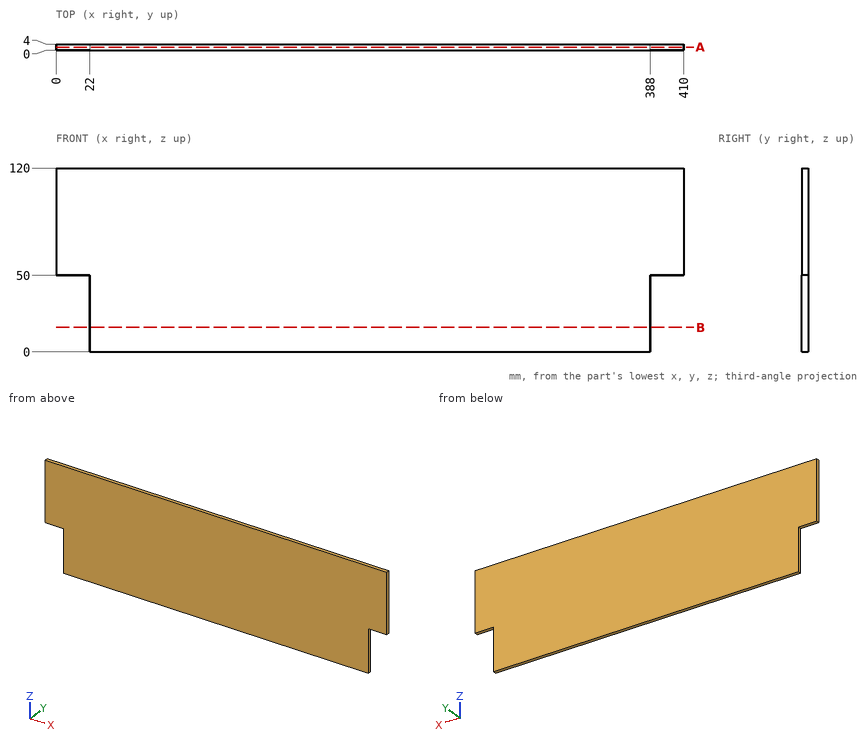
Can you work these out from the drawing? Everything is in mm from the part's minimum corner. Give positions to 0.01 mm unless a question says otherwise; leave off trailing zeros. Order: outer loops, then holes, each group sorted by start corner. A loop starts at its lowest first (then second) coordinate and runs counter-clockwise, first axis right, second up. Notation, with made-up numbers: M 22,-24 L 35,-24 A14 cw 35,2 Z; hole C -14.5,53 d4. An arc over 180 degrees is marked long. Use a Markdown table: item, result. Add a question column.
Item 1: Will these pins go through, and if not, where does the flat tip stop? pin 1 (2 mm diameter, centred on x = 402.5, y = 3, fed in from -Z); pin 2 (1.5 mm diameter, centred on y = 3.5, z = 24, fed in from -X).
Item 2: Suppose I cut it at B-B (z = 16). List the corners of the cut face in (x, y) for me.
Item 3: Suppose I cut it at A-A (y = 2). List the corners of the cut face in (x, z) for me, then the cut area to 3 significant figures.
Item 4: If I drill on L1, parallel to X at y = 2.7, z = 11.5, over which ranges is the centre line in solid material (lowest first)? Write a range as [from, to].
Answer sheet:
| question | item | result |
|---|---|---|
| 1 | pin 1 | stops at z = 50 |
| 1 | pin 2 | stops at x = 22 |
| 2 | outline | M 22,0 L 388,0 L 388,4 L 22,4 Z |
| 3 | outline | M 0,50 L 22,50 L 22,0 L 388,0 L 388,50 L 410,50 L 410,120 L 0,120 Z |
| 3 | area | 47,000 mm² |
| 4 | L1 | x = [22, 388] |
